Part model, mm, in its own coordinate system. Give positions to 0.01 mm unless a question says otherwise; leave off trailing zeros. Order: outer loops, then holes, each group sorted by start corner. A loop starts at its lowest first (then second) coordinate and runs counter-clockwise, first axis right, second up. Notation, with made-up numbers: M 64.5,9.25 L 71.5,9.25 A18 cw 71.5,42.25 Z; hole C 13.5,18 d1. An arc over 180 degrees is marked long. Return JSON: item names as keys, results as strings.
from build123d import *

# Parameters (mm, degrees)
SKETCH1_R                    = 25.4
BOSS_EXTRUDE1_DEPTH          = 3.175
F_10_0_1935_DIAMETER_HOLE1_D = 4.9149


with BuildPart() as part:
    # Sketch1 → Boss-Extrude1 (new body)
    with BuildSketch(Plane.XY):
        with BuildLine():
            Line((-115.39963726, 121.856862886), (118.175506769, 53.775916926))
            ThreePointArc((118.175506769, 53.775916926), (123.677628265, 50.487202579), (126.872726544, 44.930195291))
            Line((126.872726544, 44.930195291), (185.309252431, -168.971096981))
            ThreePointArc((185.309252431, -168.971096981), (183.152652559, -180.024636286), (173.058204177, -185.018008497))
            Line((173.058204177, -185.018008497), (-168.674542419, -185.018008497))
            ThreePointArc((-168.674542419, -185.018008497), (-178.403306847, -180.48141114), (-181.181600882, -170.112676641))
            Line((-181.181600882, -170.112676641), (-131.460524201, 111.869561592))
            ThreePointArc((-131.460524201, 111.869561592), (-125.659927441, 120.449097441), (-115.39963726, 121.856862886))
        make_face()
        with Locations((0, -121.518008497)):
            Circle(SKETCH1_R, mode=Mode.SUBTRACT)
    extrude(amount=BOSS_EXTRUDE1_DEPTH)

    # #10 (0.1935) Diameter Hole1 (through all)
    with Locations(Plane.XY.offset(3.175)):
        with Locations((-115.585524201, 103.906991503), (114.172726544, 37.231991503), (166.708204177, -165.968008497), (-162.324542419, -165.968008497)):
            Hole(F_10_0_1935_DIAMETER_HOLE1_D / 2)


solid = part.part
Q1. Band-saw the part on A-A (y = -143). Give the cut face in (x, z) (3 decimals).
Established:
{"outline": "M -176.401,0 L -13.553,0 L -13.553,3.175 L -176.401,3.175 Z; M 13.553,0 L 178.214,0 L 178.214,3.175 L 13.553,3.175 Z"}
Q2. Band-saw the part on C-C (z = 1.9). Give the cut face in (x, y).
Established:
{"outline": "M -181.18,-170.11 A12.7 ccw -168.67,-185.02 L 173.06,-185.02 A12.7 ccw 185.31,-168.97 L 126.87,44.93 A12.7 ccw 118.18,53.78 L -115.4,121.86 A12.7 ccw -131.46,111.87 Z; hole C -162.32,-165.97 d4.91; hole C -115.59,103.91 d4.91; hole C 0,-121.52 d50.8; hole C 114.17,37.23 d4.91; hole C 166.71,-165.97 d4.91"}
Q3. Probe line 1 along X through (y, z) = (-142, 2.1); line 2 along Y through (x, z) = (2.5, 0.9); line 3 along Y through (x, z) = (-26, 0.75). List the from-to ranges inside material, lowest first.
Established:
{"line 1": "x = -176.22 to -15.02, 15.02 to 177.94", "line 2": "y = -185.02 to -146.79, -96.24 to 87.49", "line 3": "y = -185.02 to 95.8"}
Q4. Band-saw the part on B-B (x = -1). Give the cut face in (y, z) (3 decimals).
Established:
{"outline": "M -185.018,0 L -146.898,0 L -146.898,3.175 L -185.018,3.175 Z; M -96.138,0 L 88.512,0 L 88.512,3.175 L -96.138,3.175 Z"}
Q5. Band-saw the part on D-D (x = -44.5). Give the cut face in (y, z) (1 decimal).
Established:
{"outline": "M -185,0 L 101.2,0 L 101.2,3.2 L -185,3.2 Z"}
Q6. Two-plate mould, pull along Y, no slides. Class faces 1 (the cylindrical face through (-5.506, -146.314, 1.565)), 2 (the flat face through (5, -63, 3.175)), 3 (the cylindrical face through (123.614, 50.552, 1.565)): +Y half, -Y half, draft (parallel to the pull), parting line (faces both ways), or undercut.
Established:
{"face 1": "undercut", "face 2": "draft", "face 3": "+Y half"}
